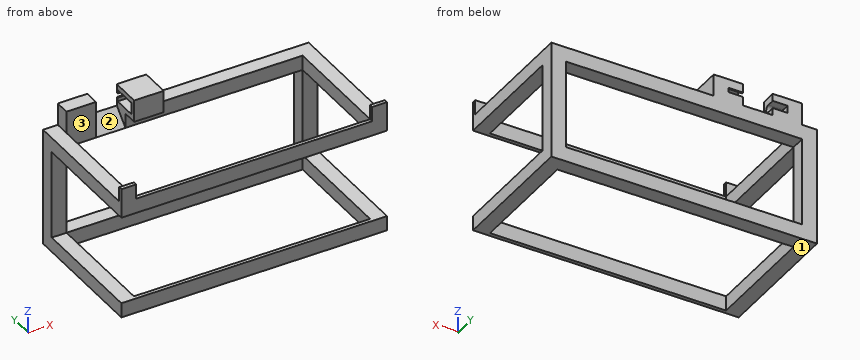
```python
from build123d import *

# Parameters (mm, degrees)
SKETCH1_W                      = 25.4
SKETCH1_H                      = 25.4
SKETCH1_W_2                    = 406.4
BOSS_EXTRUDE1_DEPTH            = 6.35
SKETCH1_4_W                    = 25.4
SKETCH1_4_H                    = 25.4
BOSS_EXTRUDE2_DEPTH            = 228.6
BOSS_EXTRUDE3_START            = 203.2
SKETCH1_5_W                    = 406.4
SKETCH1_5_H                    = 25.4
SKETCH1_5_W_2                  = 25.4
SKETCH1_5_H_2                  = 152.4
BOSS_EXTRUDE3_DEPTH            = 25.4
SKETCH2_W                      = 50.8
SKETCH2_H                      = 25.4
BOSS_EXTRUDE4_DEPTH            = 38.1
F_1_2_0_5_DIAMETER_HOLE1_D     = 12.7
F_1_2_0_5_DIAMETER_HOLE1_DEPTH = 25.4
SKETCH5_W                      = 50.8
SKETCH5_H                      = 38.1
BOSS_EXTRUDE5_DEPTH            = 25.4
SKETCH6_W                      = 20.32
SKETCH6_H                      = 40.132
CUT_EXTRUDE1_DEPTH             = 27.94
CUT_EXTRUDE2_DEPTH             = 12.7
CUT_EXTRUDE3_DEPTH             = 12.7
CUT_EXTRUDE4_START             = -76.2
CUT_EXTRUDE4_DEPTH             = 50.8


with BuildPart() as part:
    # Sketch1 → Boss-Extrude1 (new body)
    with BuildSketch(Plane(origin=(0, 0, 0), x_dir=(1, 0, 0), z_dir=(0, 1, 0))):
        with Locations((-215.9, -88.9)):
            Rectangle(SKETCH1_W, SKETCH1_H)
        with Locations((-215.9, -114.3)):
            Rectangle(SKETCH1_W, SKETCH1_H)
        with Locations((0, -88.9)):
            Rectangle(SKETCH1_W_2, SKETCH1_H)
        with Locations((215.9, -88.9)):
            Rectangle(SKETCH1_W, SKETCH1_H)
        with Locations((215.9, -114.3)):
            Rectangle(SKETCH1_W, SKETCH1_H)
        with Locations((0, 88.9)):
            Rectangle(SKETCH1_W_2, SKETCH1_H)
    extrude(amount=BOSS_EXTRUDE1_DEPTH)

    # Sketch1<4> → Boss-Extrude2 (add)
    with BuildSketch(Plane(origin=(0, 0, 0), x_dir=(1, 0, 0), z_dir=(0, 1, 0))):
        with Locations((-215.9, -88.9)):
            Rectangle(SKETCH1_4_W, SKETCH1_4_H)
        with Locations((215.9, -88.9)):
            Rectangle(SKETCH1_4_W, SKETCH1_4_H)
        with Locations((215.9, 88.9)):
            Rectangle(SKETCH1_4_W, SKETCH1_4_H)
        with Locations((-215.9, 88.9)):
            Rectangle(SKETCH1_4_W, SKETCH1_4_H)
    extrude(amount=BOSS_EXTRUDE2_DEPTH)

    # Sketch1<5> → Boss-Extrude3 (add)
    with BuildSketch(Plane(origin=(0, 0, 0), x_dir=(1, 0, 0), z_dir=(0, 1, 0)).offset(BOSS_EXTRUDE3_START)):
        with Locations((0, 88.9)):
            Rectangle(SKETCH1_5_W, SKETCH1_5_H)
        with Locations((0, -88.9)):
            Rectangle(SKETCH1_5_W, SKETCH1_5_H)
        with Locations((-215.9, 0)):
            Rectangle(SKETCH1_5_W_2, SKETCH1_5_H_2)
        with Locations((215.9, 0)):
            Rectangle(SKETCH1_5_W_2, SKETCH1_5_H_2)
    extrude(amount=BOSS_EXTRUDE3_DEPTH)

    # Sketch2 → Boss-Extrude4 (add)
    with BuildSketch(Plane.XY.offset(101.6)):
        with Locations((-177.8, 215.9)):
            Rectangle(SKETCH2_W, SKETCH2_H)
        with Locations((-76.2, 215.9)):
            Rectangle(SKETCH2_W, SKETCH2_H)
    extrude(amount=BOSS_EXTRUDE4_DEPTH)

    # 1/2 (0.5) Diameter Hole1
    with Locations(Plane(origin=(-152.4, 0, 0), x_dir=(0, 0, -1), z_dir=(1, 0, 0))):
        with Locations((-120.65, 215.9)):
            Hole(F_1_2_0_5_DIAMETER_HOLE1_D / 2, depth=F_1_2_0_5_DIAMETER_HOLE1_DEPTH)

    # Sketch5 → Boss-Extrude5 (add)
    with BuildSketch(Plane.XZ.offset(-203.2)):
        with Locations((-76.2, 120.65)):
            Rectangle(SKETCH5_W, SKETCH5_H)
    extrude(amount=BOSS_EXTRUDE5_DEPTH)

    # Sketch6 → Cut-Extrude1 (cut)
    with BuildSketch(Plane.ZY.offset(101.6)):
        with Locations((120.65, 205.994)):
            Rectangle(SKETCH6_W, SKETCH6_H)
    extrude(amount=-CUT_EXTRUDE1_DEPTH, mode=Mode.SUBTRACT)

    # Sketch7 → Cut-Extrude2 (cut)
    with BuildSketch(Plane(origin=(0, 228.6, 0), x_dir=(1, 0, 0), z_dir=(0, 1, 0))):
        Polygon((-152.4, -127), (-152.4, -114.3), (-177.8, -114.3), (-177.8, -120.65), (-177.8, -127), align=None)
    extrude(amount=-CUT_EXTRUDE2_DEPTH, mode=Mode.SUBTRACT)

    # Sketch8 → Cut-Extrude3 (cut)
    with BuildSketch(Plane(origin=(0, 228.6, 0), x_dir=(1, 0, 0), z_dir=(0, 1, 0))):
        Polygon((-101.6, -124.46), (-76.2, -124.46), (-76.2, -120.65), (-76.2, -116.84), (-101.6, -116.84), (-101.6, -120.65), align=None)
    extrude(amount=-CUT_EXTRUDE3_DEPTH, mode=Mode.SUBTRACT)

    # Sketch9 → Cut-Extrude4 (cut)
    with BuildSketch(Plane.ZY.offset(228.6).offset(CUT_EXTRUDE4_START)):
        Polygon((76.2, 203.2), (101.6, 228.6), (101.6, 203.2), align=None)
    extrude(amount=-CUT_EXTRUDE4_DEPTH, mode=Mode.SUBTRACT)


solid = part.part
```
Source: CAD feature listing. Evaluate the final solid. Frame: model axes, mm. Face numbers are marked on the shaded views. Coordinates: 2 decimals unless noted, no trailing zeros. Write each loop counter-clockwise with the first axis right and the second up, starting at its lowest first coordinate (ties: lowest second). Pieces come first, ordered by that corner, then holes. Notation, with made-up numbers: M 42.5,8.25 L 86.5,8.25 A26 cw 86.5,23.25 Z; hole C -22,-30 d8. An arc over 180 degrees is marked long. Answer as a JSON object with one key per item and string values.
1. Cut plane B-B on y = 15. Output: boundary loops of the cut face in (x, z).
Evaluation:
{"outline": "M -228.6,-101.6 L -203.2,-101.6 L -203.2,-76.2 L -228.6,-76.2 Z; M -228.6,76.2 L -203.2,76.2 L -203.2,101.6 L -228.6,101.6 Z; M 203.2,-101.6 L 228.6,-101.6 L 228.6,-76.2 L 203.2,-76.2 Z; M 203.2,76.2 L 228.6,76.2 L 228.6,101.6 L 203.2,101.6 Z"}
2. Cut plane C-C on z = -64. Output: boundary loops of the cut face in (x, y), plus the area to 3 significant figures.
Evaluation:
{"outline": "M -228.6,203.2 L -203.2,203.2 L -203.2,228.6 L -228.6,228.6 Z; M 203.2,203.2 L 228.6,203.2 L 228.6,228.6 L 203.2,228.6 Z", "area": "1,290 mm^2"}
3. Contact query for flat-ended pins moving along their axis: P1, Ø20.5, axis at x = 38, y = 211.5, coming from the +Z side; P2, Ø5, axis at x = 212, y = 2.5, coming from the +Z side; P3, Ø6, axis at y = 200.5, z = 120, coming from the -X side. Output: stop coordinate, or through.
Evaluation:
{"P1": "z = 101.6", "P2": "z = 127", "P3": "x = -203.2"}
4. Cut plane A-A on x = -60. Output: boundary loops of the cut face in (y, z), plus the area to 3 significant figures.
Evaluation:
{"outline": "M 0,-101.6 L 6.35,-101.6 L 6.35,-76.2 L 0,-76.2 Z; M 0,76.2 L 6.35,76.2 L 6.35,101.6 L 0,101.6 Z; M 177.8,101.6 L 203.2,101.6 L 203.2,76.2 L 228.6,76.2 L 228.6,139.7 L 177.8,139.7 Z; M 203.2,-101.6 L 228.6,-101.6 L 228.6,-76.2 L 203.2,-76.2 Z", "area": "3,550 mm^2"}
5. Ray query, L1, parallel to Z at x = -23.5, y = 205; L2, parallel to X at y = 205.5, z = 64; L3, parallel to Y at x = -48.5, z = -83. Return the intervals inside material, ascending.
Evaluation:
{"L1": "-101.6 to -76.2, 76.2 to 101.6", "L2": "-228.6 to -203.2, 203.2 to 228.6", "L3": "0 to 6.35, 203.2 to 228.6"}
6. Draft query along X for the marked faces 1, 2 and 3. Return one class per face: released by +X, released by -X, zero draft, split by the parting line, or undercut.
Evaluation:
{"face 1": "zero draft", "face 2": "undercut", "face 3": "undercut"}
7. Cut plane D-D on x = 93. Output: boundary loops of the cut face in (y, z).
Evaluation:
{"outline": "M 0,-101.6 L 6.35,-101.6 L 6.35,-76.2 L 0,-76.2 Z; M 0,76.2 L 6.35,76.2 L 6.35,101.6 L 0,101.6 Z; M 203.2,-101.6 L 228.6,-101.6 L 228.6,-76.2 L 203.2,-76.2 Z; M 203.2,76.2 L 228.6,76.2 L 228.6,101.6 L 203.2,101.6 Z"}
